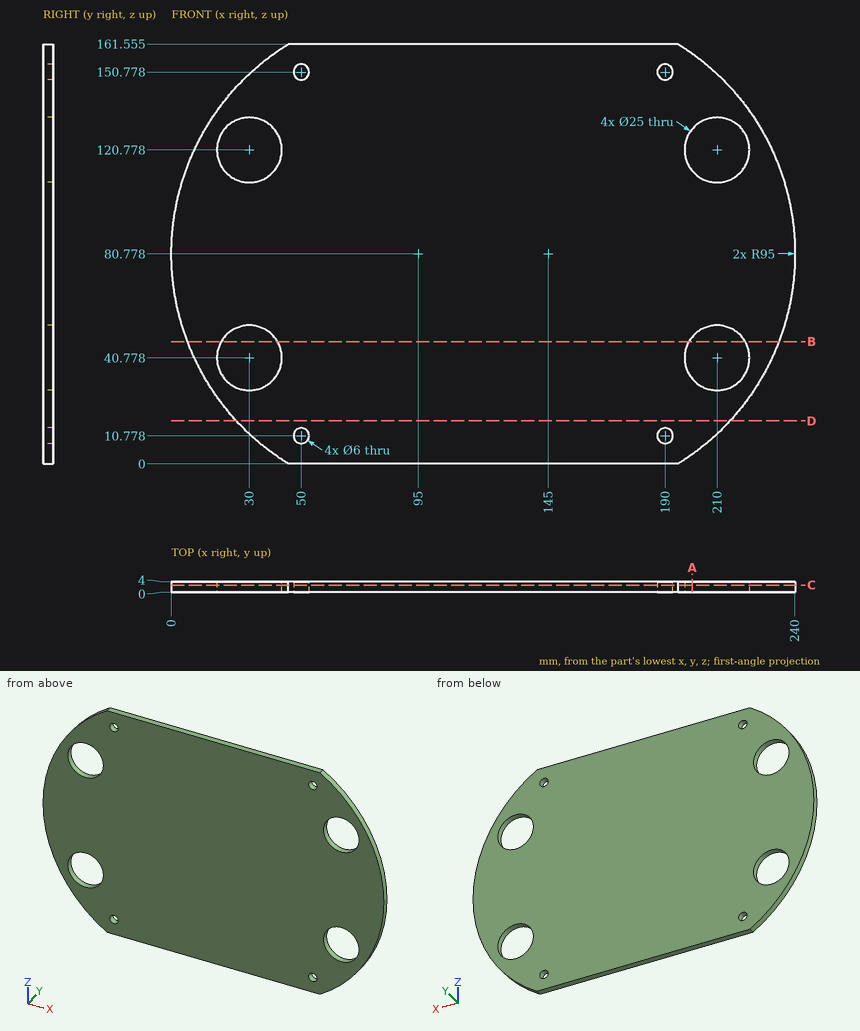
Here's the drawing with two shaded views (mm, measured from the low corner). I have some questions. Give positions to 0.01 mm unless a question says otherwise; leave off trailing zeros. Loops run counter-clockwise (first coordinate to the right, second up) from the corner with the lowest first, then second, coordinate; pieces in that order, holes last. Notation, with made-up numbers: M 70.5,-2 L 117.5,-2 A17 cw 117.5,18 Z; hole C 45,-14 d11. An arc over 180 degrees is marked long. One line per item, written item: value. Start each with the question number.
1) If we section it at D-D, the plane z = 16.5: Write out the boundary of the cut face in (x, y).
2) If we section it at A-A, the plane x = 200.5: Write out the boundary of the cut face in (y, z) (1 decimal).
3) If I drill on line 1 (X direction, y = 2.4, z = 114.5) (1 decimal); line 2 (X direction, y = 2.9, z = 118) (1 decimal); line 3 (Z direction, x = 191.5, y = 0.95) (1 decimal), over which ranges is the centre line in solid material (lowest first)? Write a range as [from, to].
4) If we section it at B-B, the plane z = 47: Write out the boundary of the cut face in (x, y).
5) If we section it at C-C, the plane y = 2.75: Give the number of separate pieces and of enclosed holes in the cut face, and give its area (3 significant figures).
6) I'm going to push flat-ended pins straight in: pin 1 (1.5 mm diameter, centred on y = 0.5, z = 37.5, fed in from -X); pin 2 (2 mm diameter, centred on y = 2, z = 113.5, fed in from -X); pin 3 (2 mm diameter, centred on y = 2.5, z = 65, fed in from +X). Where does each tip first touch, or does it pass through?
Completed:
1. outline: M 25.05,0 L 214.95,0 L 214.95,4 L 25.05,4 Z
2. outline: M 0,3.7 L 4,3.7 L 4,32.7 L 0,32.7 Z; M 0,48.9 L 4,48.9 L 4,112.7 L 0,112.7 Z; M 0,128.9 L 4,128.9 L 4,157.9 L 0,157.9 Z
3. line 1: x = [6.2, 19.2], [40.8, 199.2], [220.8, 233.8]
3. line 2: x = [7.6, 17.8], [42.2, 197.8], [222.2, 232.4]
3. line 3: z = [0, 8.2], [13.4, 148.2], [153.4, 161.6]
4. outline: M 6.21,0 L 19.16,0 L 19.16,4 L 6.21,4 Z; M 40.84,0 L 199.16,0 L 199.16,4 L 40.84,4 Z; M 220.84,0 L 233.79,0 L 233.79,4 L 220.84,4 Z
5. separate pieces: 1
5. enclosed holes: 8
5. area: 32,400 mm^2
6. pin 1: stops at x = 10.05
6. pin 2: stops at x = 5.45
6. pin 3: stops at x = 238.84
